For this review, take the finished solid that the model builds, in its own axes (mm). A direction names the side the tool comes from. Give positions to 0.01 mm unless a question says otherwise; leave off trailing zeros. Order: outer loops, then holes, each group sorted by start corner. A loop starts at its lowest first (then second) coordinate and runs counter-clockwise, first axis right, second up.
from build123d import *

# Parameters (mm, degrees)
F0_W     = 125
F0_H     = 52
F0_R     = 1.785938
F0_R_2   = 1.5875
F1_DEPTH = 5.5


with BuildPart() as f1:
    # F0 (on Front) → F1 (new body)
    with BuildSketch(Plane.XZ):
        with Locations((62.5, 26)):
            Rectangle(F0_W, F0_H)
        with Locations((111, 14)):
            Circle(F0_R, mode=Mode.SUBTRACT)
        Polygon((58.416788, 31.5), (58.416788, 26), (58.416788, 20.5), (36.416788, 20.5), (36.416788, 31.5), align=None, mode=Mode.SUBTRACT)
        with Locations((82.416788, 26)):
            Circle(F0_R_2, mode=Mode.SUBTRACT)
    extrude(amount=F1_DEPTH)


solid = f1.part
1) We need section A-A on x = 111. Give the boundary of the cut face in (y, z), then the cut area to 3 significant figures.
Answer sheet:
outline: (-5.5, 0) - (0, 0) - (0, 12.21) - (-5.5, 12.21) - close; (-5.5, 15.79) - (0, 15.79) - (0, 52) - (-5.5, 52) - close
area: 266 mm2
2) Draft analysis for pull direction X (two halves, no side actions). For faces 3 (the face through (62, -3, 0)), 4 (the face through (36.417, -3, 26)), 5 (the face through (0, -3, 26)), 6 (the face through (125, -3, 26)), state which applies: +X half, -X half, draft (parallel to the pull), parting line (faces both ways), or undercut.
Answer sheet:
face 3: draft
face 4: undercut
face 5: -X half
face 6: +X half
3) Tool access review of faces 1 (the face through (62, 0, 26)), 2 (the face through (47, -3, 31.5)): name each direction out of +Z, -Z, +X, -X, +Y, -Y from which nothing blocks a thin tool from reaching the whole face with its end or side.
Answer sheet:
face 1: +Z, -Z, +X, -X, +Y
face 2: +Y, -Y
4) To check wall thickness, follow line 1 (X direction, y = -1.35, z = 22.5); line 2 (Z direction, x = 111, y = -3.25); line 3 (Z direction, x = 47, y = -1.9). State the ranges of each line that lie inside material, in increasing order.
Answer sheet:
line 1: x = 0 to 36.42, 58.42 to 125
line 2: z = 0 to 12.21, 15.79 to 52
line 3: z = 0 to 20.5, 31.5 to 52
5) We need section B-B on z = 29.5. Give the boundary of the cut face in (x, y).
Answer sheet:
outline: (0, -5.5) - (36.42, -5.5) - (36.42, 0) - (0, 0) - close; (58.42, -5.5) - (125, -5.5) - (125, 0) - (58.42, 0) - close
6) We need section C-C on y = -2.6. Give the boundary of the cut face in (x, z) (1 decimal).
Answer sheet:
outline: (0, 0) - (125, 0) - (125, 52) - (0, 52) - close; hole (36.4, 20.5) - (58.4, 20.5) - (58.4, 31.5) - (36.4, 31.5) - close; hole circle Ø3.2 at (82.4, 26); hole circle Ø3.6 at (111, 14)
7) Clearance check with a flat-ended pin moving along its axis: pin 1 (3 mm diameter, centred on x = 111, z = 14, fed in from +Y). State where the tip first meets the part, or that it passes through.
Answer sheet:
pin 1: passes through
